For this review, take the finished solid that the model builds, in its own axes (mm). A direction names the side the tool comes from. Give positions to 0.01 mm unless a question says otherwise; leave off trailing zeros. Write each loop counter-clockwise with the first axis right and the second up, starting at its lowest first coordinate (ties: lowest second). Pieces come first, ordered by that corner, then holes.
Q1. Insertion check: P1, Ø5, axis at x = 10.14, y = 5.71, coming from the +Z side; P2, Ø3, axis at x = -10.14, y = -5.71, coming from the +Z side; P3, Ø1, axis at x = -17.5, z = 1, coming from the -Y side; P4, Ø1.5, axis at x = -21.5, z = 1, coming from the -Y side. Each pin has a flat end and moves straight along its axis. Give the tip position at first contact, or say it passes through.
Q2. We need section D-D (y = 18.54). Write out the cut boundary in (x, z).
Q3. Machinability: for faces 5 (the flat face through (-8, -2.55, 2)), 6 (the flat face through (23.71, 46.24, 1.56)), which of the approach directions +Z, -Z, +X, -X, +Y, -Y give a long, thin tool a straight path to every point of the face, cutting with its end or side? Answer none if there is none.
Q4. We need section C-C (z = 1.8). Give the number of separate pieces and of enclosed holes in the cut face, then the cut area to 3 significant figures.
Q5. Mouldability with a two-part tool opening along X and no side actions: class faces 1 (the cylindrical face through (7.065, -0.274, 1.563)), 2 (the flat face through (48.9, 8.8, 1.6)), 3 (the flat face through (14, 9, 3.17)), 4 (the cylindrical face through (64.495, 50.446, 1.563)) as released by +X, released by -X, zero draft, split by the parting line, or undercut.
Q6. For line 1 (X direction, y = 6.5, z = 0.25); line 2 (Y direction, x = -10.14, z = 0.75); line 3 (X direction, y = -1, z = 1.7), list the stretches that pass through material, from the lowest coordinate up.
Q7. We need section B-B (x = 18.54). Write out the cut boundary in (y, z).
Q8. We need section A-A (y = -5.71). Write out the cut boundary in (x, z), then the cut area to 3 significant figures.
```python
from build123d import *

# Parameters (mm, degrees)
SKETCH1_R             = 7.07
BOSS_EXTRUDE2_DEPTH   = 3.17
SKETCH2_R             = 1.799813297
CUT_EXTRUDE1_DEPTH    = 3.17
CIRPATTERN1_COUNT     = 4
F_4_0MM_DOWEL_HOLE1_D = 4
CIRPATTERN2_COUNT     = 6
CUT_EXTRUDE2_REACH    = 88.731


with BuildPart() as part:
    # Sketch1 → Boss-Extrude2 (new body)
    # profile 1 of 2: a face of its own
    with BuildSketch(Plane.XY):
        with BuildLine():
            ThreePointArc((-5.13430178, 37.651546386), (-31.529571408, -21.210519249), (32.94, -18.946144727))
            ThreePointArc((32.94, -18.946144727), (36.71321288, -9.805100713), (38, 0))
            ThreePointArc((38, 0), (24.988962887, 28.62781399), (-5.13430178, 37.651546386))
        make_face()
        Circle(SKETCH1_R, mode=Mode.SUBTRACT)
    # profile 2 of 2: a face of its own
    with BuildSketch(Plane.XY):
        with BuildLine():
            ThreePointArc((38, 0), (36.71321288, -9.805100713), (32.94, -18.946144727))
            Line((32.94, -18.946144727), (65.347879138, 37.398592116))
            ThreePointArc((65.347879138, 37.398592116), (64.374631715, 50.601425699), (51.751457407, 54.591099312))
            Line((51.751457407, 54.591099312), (-5.13430178, 37.651546386))
            ThreePointArc((-5.13430178, 37.651546386), (24.988962887, 28.62781399), (38, 0))
        make_face()
    extrude(amount=BOSS_EXTRUDE2_DEPTH)

    # Sketch2 → Cut-Extrude1 (cut)
    with BuildSketch(Plane.XY.offset(3.17)):
        with Locations((-18.54, 0)):
            Circle(SKETCH2_R)
    cut_extrude1 = extrude(amount=-CUT_EXTRUDE1_DEPTH, mode=Mode.SUBTRACT)

    # CirPattern1: Cut-Extrude1 ×4 about axis
    cirpattern1_axis = Axis((0, 0, 0), (0, 0, 1))
    for i in range(1, CIRPATTERN1_COUNT):
        add(cut_extrude1.rotate(cirpattern1_axis, i * 360 / CIRPATTERN1_COUNT), mode=Mode.SUBTRACT)

    # Ø4.0mm Dowel Hole1 (through all)
    with Locations(Plane.XY.offset(3.17)):
        with Locations((-10.14, -5.71)):
            f_4_0mm_dowel_hole1 = Hole(F_4_0MM_DOWEL_HOLE1_D / 2)

    # CirPattern2: Ø4.0mm Dowel Hole1 ×6 about axis
    cirpattern2_axis = Axis((0, 0, 0), (0, 0, 1))
    for i in range(1, CIRPATTERN2_COUNT):
        add(f_4_0mm_dowel_hole1.rotate(cirpattern2_axis, i * 360 / CIRPATTERN2_COUNT), mode=Mode.SUBTRACT)

    # Sketch5 → Cut-Extrude2 (cut, up to next)
    with BuildSketch(Plane(origin=(0, 0, 0), x_dir=(-1, 0, 0), z_dir=(0, 0, -1)), mode=Mode.PRIVATE) as cut_extrude2_sk1:
        with BuildLine():
            Line((6.594118592, 2.55), (9.57, 2.55))
            Line((9.57, 2.55), (9.57, -2.55))
            Line((9.57, -2.55), (6.594118592, -2.55))
            ThreePointArc((6.594118592, -2.55), (7.07, 0), (6.594118592, 2.55))
        make_face()
    cut_extrude2_tool1 = extrude(cut_extrude2_sk1.sketch, amount=-CUT_EXTRUDE2_REACH, mode=Mode.PRIVATE) & part.part
    add(cut_extrude2_tool1.solids().sort_by_distance((-8.238036, 0, 0))[0], mode=Mode.SUBTRACT)


solid = part.part
```
Computed:
1. P1: stops at z = 3.17
1. P2: passes through
1. P3: stops at y = -33.99
1. P4: stops at y = -31.83
2. outline: (-33.17, 0) - (-1.8, 0) - (-1.8, 3.17) - (-33.17, 3.17) - close; (1.8, 0) - (54.5, 0) - (54.5, 3.17) - (1.8, 3.17) - close
3. face 5: +Z, -Z
3. face 6: +Z, -Z, -X, +Y
4. separate pieces: 1
4. enclosed holes: 11
4. area: 5,920 mm2
5. face 1: undercut
5. face 2: released by +X
5. face 3: zero draft
5. face 4: split by the parting line
6. line 1: x = -37.44 to -11.93, -8.1 to -2.78, 2.78 to 8.3, 11.98 to 47.58
6. line 2: y = -36.62 to -7.71, -3.71 to 3.93, 7.92 to 36.62
6. line 3: x = -37.99 to -20.04, -17.04 to -9.57, 7 to 17.04, 20.04 to 43.26
7. outline: (-33.17, 0) - (-1.8, 0) - (-1.8, 3.17) - (-33.17, 3.17) - close; (1.8, 0) - (44.7, 0) - (44.7, 3.17) - (1.8, 3.17) - close
8. outline: (-37.57, 0) - (-12.14, 0) - (-12.14, 3.17) - (-37.57, 3.17) - close; (-8.14, 0) - (-4.17, 0) - (-4.17, 3.17) - (-8.14, 3.17) - close; (4.17, 0) - (8.03, 0) - (8.03, 3.17) - (4.17, 3.17) - close; (12, 0) - (40.55, 0) - (40.55, 3.17) - (12, 3.17) - close
8. area: 196 mm2
